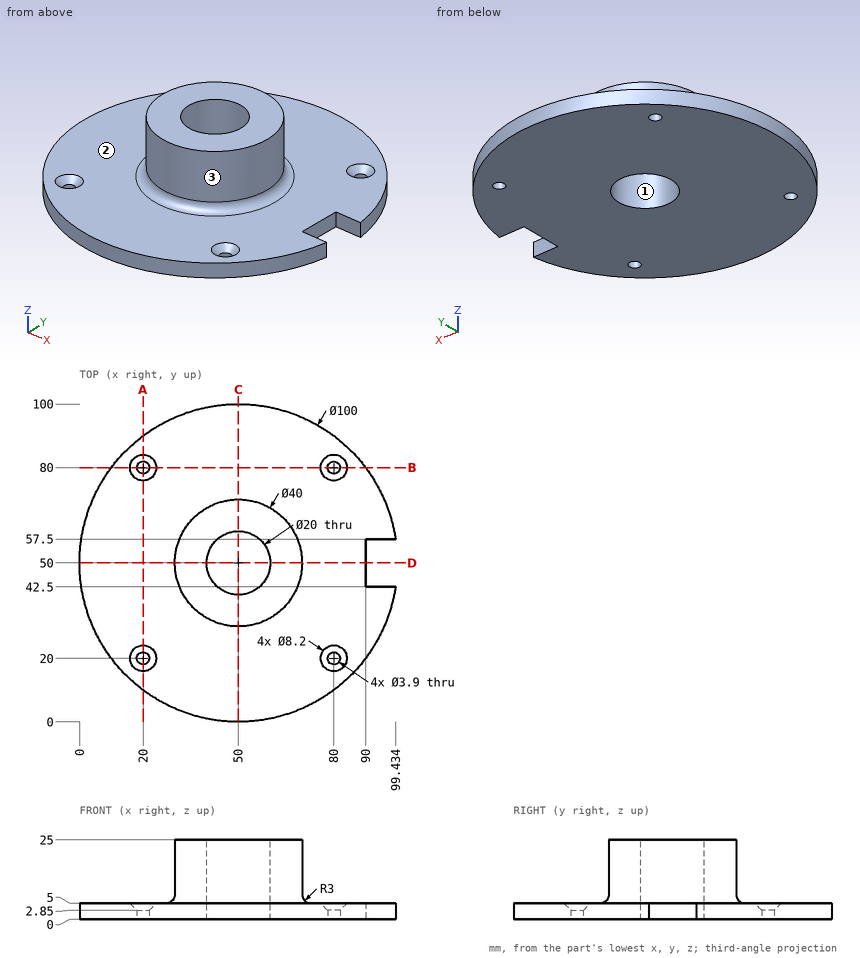
Check sheet for the drawn part. Datum: minimum x, y, z corner. Units: mm. Give positions to 0.01 mm unless a question says otherwise; leave off trailing zeros. Order: outer loops, then holes, each group sorted by start corner. A loop starts at its lowest first (then second) coordinate and runs counter-clockwise, first axis right, second up. Notation, with made-up numbers: (45, 57.25) -> (81, 57.25) arc R18 cw to (81, 61.25) -> close; hole circle Ø9 at (-15.5, 11). An arc over 180 degrees is marked (long way). One line per item, written item: value.
(1) Draft check along X on the marked faces 1, 2 and 3. Enter one of: pulls with the +X half, pulls with the -X half, needs draft (parallel to the pull), parting line crosses it, or undercut.
Final values:
face 1: undercut
face 2: needs draft
face 3: parting line crosses it
(2) Sectioned sample at D-D on y = 50. Record the cut outline in (x, z), then the cut area to 3 significant figures.
Final values:
outline: (0, 0) -> (40, 0) -> (40, 25) -> (30, 25) -> (30, 8) arc R3 cw to (27, 5) -> (0, 5) -> close; (60, 0) -> (90, 0) -> (90, 5) -> (73, 5) arc R3 cw to (70, 8) -> (70, 25) -> (60, 25) -> close
area: 754 mm^2
(3) Sectioned sample at A-A on x = 20. Record the cut outline in (y, z), then the cut area to 3 significant figures.
Final values:
outline: (10, 0) -> (18.05, 0) -> (18.05, 2.85) -> (15.9, 5) -> (10, 5) -> close; (21.95, 0) -> (78.05, 0) -> (78.05, 2.85) -> (75.9, 5) -> (24.1, 5) -> (21.95, 2.85) -> close; (81.95, 0) -> (90, 0) -> (90, 5) -> (84.1, 5) -> (81.95, 2.85) -> close
area: 352 mm^2
(4) Sectioned sample at C-C on x = 50. Record the cut outline in (y, z), then the cut area to 3 significant figures.
Final values:
outline: (0, 0) -> (40, 0) -> (40, 25) -> (30, 25) -> (30, 8) arc R3 cw to (27, 5) -> (0, 5) -> close; (60, 0) -> (100, 0) -> (100, 5) -> (73, 5) arc R3 cw to (70, 8) -> (70, 25) -> (60, 25) -> close
area: 804 mm^2
(5) Gauge pin test, flat ends, axial feed: pin 1 (5.5 mm diameter, centred on y = 47.5, z = 3.5, fed in from +X); pin 2 (2 mm diameter, centred on y = 33, z = 19, fed in from -X); pin 3 (2 mm diameter, centred on x = 23, z = 3, fed in from -Y); pin 4 (8 mm diameter, centred on y = 60.5, z = 5, fed in from +X). Record the tip position at first contact, or that the pin passes through.
Final values:
pin 1: x = 90
pin 2: x = 38
pin 3: y = 7.29
pin 4: x = 99.43
(6) Scan lines: line 1 along X through (y, z) = (20, 1.8); line 2 along Y through (x, z) = (21, 4.75); line 3 along Z through (x, y) = (85, 25.5). Record each from-to range of solid material in increasing order. Write a range as [from, to].
Final values:
line 1: [10, 18.05], [21.95, 78.05], [81.95, 90]
line 2: [9.27, 16.28], [23.72, 76.28], [83.72, 90.73]
line 3: [0, 5]
